Read the model definition and answer for the solid it produces. Units are mm, in the model's axes. A direction names the side the tool comes from. Coordinates: 2 decimals unless noted, no trailing zeros. Order: outer loops, then holes, each group sorted by start corner. A loop starts at its lowest first (then second) coordinate and runs counter-clockwise, first axis right, second up. Notation, with made-up numbers: (-37, 88.25) -> (-10, 88.25) arc R19 ccw to (-10, 108.25) -> close; hole circle Ø7 at (85.25, 29). An arc over 180 degrees is marked (long way). Answer in a Markdown table with one row per item.
from build123d import *

# Parameters (mm, degrees)
BOSS_EXTRUDE1_DEPTH = 20
SKETCH3_W           = 15
SKETCH3_H           = 20
CUT_EXTRUDE1_DEPTH  = 10
SKETCH4_W           = 15
SKETCH4_H           = 20
CUT_EXTRUDE2_DEPTH  = 10


with BuildPart() as part:
    # Sketch1 → Boss-Extrude1 (new body)
    with BuildSketch(Plane(origin=(0, 0, 0), x_dir=(1, 0, 0), z_dir=(0, 1, 0))):
        with BuildLine():
            Line((-10, 30), (-10, 270))
            ThreePointArc((-10, 270), (1.715728753, 298.284271247), (30, 310))
            Line((30, 310), (190, 310))
            ThreePointArc((190, 310), (218.284271247, 298.284271247), (230, 270))
            Line((230, 270), (230, 30))
            ThreePointArc((230, 30), (218.284271247, 1.715728753), (190, -10))
            Line((190, -10), (30, -10))
            ThreePointArc((30, -10), (1.715728753, 1.715728753), (-10, 30))
        make_face()
    extrude(amount=BOSS_EXTRUDE1_DEPTH)

    # Sketch3 → Cut-Extrude1 (cut)
    with BuildSketch(Plane.ZY.offset(10)):
        with Locations((-247.5, 10)):
            Rectangle(SKETCH3_W, SKETCH3_H)
        with Locations((-217.5, 10)):
            Rectangle(SKETCH3_W, SKETCH3_H)
        with Locations((-187.5, 10)):
            Rectangle(SKETCH3_W, SKETCH3_H)
        with Locations((-157.5, 10)):
            Rectangle(SKETCH3_W, SKETCH3_H)
        with Locations((-127.5, 10)):
            Rectangle(SKETCH3_W, SKETCH3_H)
        with Locations((-97.5, 10)):
            Rectangle(SKETCH3_W, SKETCH3_H)
        with Locations((-67.5, 10)):
            Rectangle(SKETCH3_W, SKETCH3_H)
        with Locations((-37.5, 10)):
            Rectangle(SKETCH3_W, SKETCH3_H)
    extrude(amount=-CUT_EXTRUDE1_DEPTH, mode=Mode.SUBTRACT)

    # Sketch4 → Cut-Extrude2 (cut)
    with BuildSketch(Plane(origin=(230, 0, 0), x_dir=(0, 0, -1), z_dir=(1, 0, 0))):
        with Locations((247.5, 10)):
            Rectangle(SKETCH4_W, SKETCH4_H)
        with Locations((217.5, 10)):
            Rectangle(SKETCH4_W, SKETCH4_H)
        with Locations((157.5, 10)):
            Rectangle(SKETCH4_W, SKETCH4_H)
        with Locations((127.5, 10)):
            Rectangle(SKETCH4_W, SKETCH4_H)
        with Locations((97.5, 10)):
            Rectangle(SKETCH4_W, SKETCH4_H)
        with Locations((67.5, 10)):
            Rectangle(SKETCH4_W, SKETCH4_H)
        with Locations((37.5, 10)):
            Rectangle(SKETCH4_W, SKETCH4_H)
        with Locations((187.5, 10)):
            Rectangle(SKETCH4_W, SKETCH4_H)
    extrude(amount=-CUT_EXTRUDE2_DEPTH, mode=Mode.SUBTRACT)


solid = part.part
Q1. The part is cut by section A-A (z = -213.5). Write down the section's boundary in (x, y).
Outcome:
| item | result |
|---|---|
| outline | (0, 0) -> (220, 0) -> (220, 20) -> (0, 20) -> close |
Q2. For a pull along Z with two mould halves and no side action, classify faces 1 (the face through (225, 10, -120)), 2 (the face through (2.028, 9.86, -1.406)), 3 (the face through (0, 10, -218)), 4 (the face through (230, 10, -83)) as pulls with the +Z half, pulls with the -Z half, needs draft (parallel to the pull), parting line crosses it, or undercut.
Outcome:
| item | result |
|---|---|
| face 1 | undercut |
| face 2 | pulls with the +Z half |
| face 3 | undercut |
| face 4 | needs draft |
Q3. Given pin 1 (11 mm diameter, centred on x = 223, y = 12, fed in from +Z); pin 2 (3 mm diameter, centred on x = 227.5, y = 9, fed in from -Z); pin 3 (5 mm diameter, centred on x = -3, y = 12.5, fed in from +Z), each flat-ended and moving along its own axis, determine where each tip first touches the part or whether it passes through.
Outcome:
| item | result |
|---|---|
| pin 1 | z = -0.95 |
| pin 2 | z = -287.44 |
| pin 3 | z = -4.12 |
Q4. For faces 5 (the face through (-5, 10, -105)), 6 (the face through (220, 10, -97)), 7 (the face through (-10, 10, -232)), determine the directions among +Z, -Z, +X, -X, +Y, -Y from which every point of the face is accessible in a straight line to the end or side of a thin tool.
Outcome:
| item | result |
|---|---|
| face 5 | -X, +Y, -Y |
| face 6 | +X, +Y, -Y |
| face 7 | +Z, -Z, -X, +Y, -Y |
Q5. Consider line 1 (X direction, y = 6.5, z = -250); line 2 (X direction, y = 3, z = -283.5); line 3 (Z direction, x = 216, y = 8). Determine where each line is inside the solid, lowest interval first.
Outcome:
| item | result |
|---|---|
| line 1 | 0 to 220 |
| line 2 | -7.65 to 227.65 |
| line 3 | -300.4 to 0.4 |
